```python
from build123d import *

# Parameters (mm, degrees)
F0_R     = 22.5
F1_DEPTH = 15
F4_R     = 30
F5_DEPTH = 5
F6_R     = 15
F7_DEPTH = 35
F8_R     = 7.5
F9_DEPTH = 15


with BuildPart() as f1:
    # F0 (on Top) → F1 (new body)
    with BuildSketch(Plane.XY):
        Circle(F0_R)
    extrude(amount=F1_DEPTH)

    # F2 (on Front) → F3 (revolve)
    with BuildSketch(Plane.XZ):
        Polygon((-30, 15), (0, 15), (0, 30), (-15, 30), align=None)
    revolve(axis=Axis((0, 0, 7.5), (0, 0, 1)))

    # F4 (on face) → F5 (join)
    with BuildSketch(Plane(origin=(0, 0, 15), x_dir=(1, 0, 0), z_dir=(0, 0, -1))):
        Circle(F4_R)
    extrude(amount=F5_DEPTH)

    # F6 (on face) → F7 (join)
    with BuildSketch(Plane.XY.offset(30)):
        Circle(F6_R)
    extrude(amount=F7_DEPTH)

    # F8 (on face) → F9 (join)
    with BuildSketch(Plane.XY.offset(65)):
        Circle(F8_R)
    extrude(amount=F9_DEPTH)


solid = f1.part
```
Geometry check sheet. Reference: the model listing, model coordinates, mm. A direction names the side the tool comes from. Round coordinates to 2 decimals unless told otherwise and drop trailing zeros. Loops run counter-clockwise (first coordinate to the right, second up) from the corner with the lowest first, then second, coordinate; pieces in that order, holes last. Notation, with made-up numbers: (77.25, 50.25) - (97.25, 50.25) arc R13 ccw to (97.25, 54.25) - close; hole circle Ø3 at (-28.75, -9). An arc over 180 degrees is marked (long way). Write item = value, one per line. Start each with the question number.
1. Depth check by flat-ended pin: pin 1 (1.5 mm diameter, centred on x = -14.5, y = -6.5, fed in from +Z); pin 2 (12 mm diameter, centred on y = 11.5, z = 49, fed in from +X); pin 3 (10 mm diameter, centred on x = -14, z = 45, fed in from -Y). Enter the tip coordinate at first touch or a pass-through.
2. Set-up check for faces 1 (the face through (10.382, -19.961, 4.93)), 2 (the face through (0, 0, 0)), 3 (the face through (-14.985, 0.66, 47.255)): record each of +Z, -Z, +X, -X, +Y, -Y from which the full face is reachable in a straight line by a thin tool's end or side.
3. Section check D-D on z = 31.5. Enter the section's corners in (x, y).
4. Section check A-A on x = 0. Enter the section's corners in (y, z).
5. Section check C-C on z = 67. Enter the section's corners in (x, y), then the cut area to 3 significant figures.
6. Thickness scan on line 1 (Z direction, x = 8.5, y = -7); line 2 (X direction, y = -17, z = 5); line 3 (Y direction, x = 5, z = 61.5). Record the ranges inside material, lowest first.
Working result:
q1.pin_1 = 29.86
q1.pin_2 = 13.96
q1.pin_3 = -12
q2.face_1 = -Z
q2.face_2 = -Z, +X, -X, +Y, -Y
q2.face_3 = +Z
q3.outline = circle Ø30 at (0, 0)
q4.outline = (-30, 10) - (-22.5, 10) - (-22.5, 0) - (22.5, 0) - (22.5, 10) - (30, 10) - (30, 15) - (15, 30) - (15, 65) - (7.5, 65) - (7.5, 80) - (-7.5, 80) - (-7.5, 65) - (-15, 65) - (-15, 30) - (-30, 15) - close
q5.outline = circle Ø15 at (0, 0)
q5.area = 177 mm^2
q6.line_1 = 0 to 65
q6.line_2 = -14.74 to 14.74
q6.line_3 = -14.14 to 14.14
